Input: part model. Units: mm. Frame: model coordinates. A direction names the side the tool comes from. Give positions to 0.01 mm unless a question says otherwise; leave off trailing zeros. Loops run counter-clockwise (first coordinate to the right, second up) from the corner with the lowest first, then second, coordinate; pieces in that order, holes last. Notation, with made-up numbers: M 7.25,-8 L 22.25,-8 A17 cw 22.25,8 Z; hole C -3,-9 d10. An arc over 180 degrees is marked long. Return JSON: item names as keys, results as strings. Group by question number.
```python
from build123d import *

# Parameters (mm, degrees)
F0_R     = 4.09
F1_DEPTH = 2.6
F2_R     = 5.5
F3_DEPTH = 0.7
F4_R     = 10.95
F5_DEPTH = 1.3
F6_W     = 1.967797
F6_H     = 3.211017
F7_DEPTH = 1


with BuildPart() as f1:
    # F0 (on Top) → F1 (new body)
    with BuildSketch(Plane.XY):
        Circle(F0_R)
    extrude(amount=F1_DEPTH)

    # F2 (on face) → F3 (join)
    with BuildSketch(Plane.XY.offset(2.6)):
        Circle(F2_R)
    extrude(amount=F3_DEPTH)

    # F4 (on face) → F5 (join)
    with BuildSketch(Plane.XY.offset(3.3)):
        Circle(F4_R)
    extrude(amount=F5_DEPTH)

    # F6 (on face) → F7 (cut)
    with BuildSketch(Plane.XY.offset(4.6)):
        Polygon((-9.000013, -5.514394), (-6.681369, -5.514394), (-6.681369, -1.891513), (-4.713572, -1.891513), (-4.713572, -5.514394), (-2.402555, -5.514394), (-2.402555, 5.514419), (-7.222894, 5.514419), (-9.000013, 3.767809), align=None)
        with Locations((-5.69747, 1.811453)):
            Rectangle(F6_W, F6_H, mode=Mode.SUBTRACT)
        Polygon((-1.372894, 5.514419), (-1.372894, -5.514394), (4.172021, -5.514394), (4.172021, -3.424564), (0.938123, -3.424564), (0.938123, 5.514419), align=None)
        Polygon((8.999987, -5.514394), (8.999987, -3.424564), (8.237275, -3.424564), (8.237275, 3.424589), (8.999987, 3.424589), (8.999987, 5.514419), (5.163547, 5.514419), (5.163547, 3.424589), (5.926259, 3.424589), (5.926259, -3.424564), (5.163547, -3.424564), (5.163547, -5.514394), align=None)
    extrude(amount=-F7_DEPTH, mode=Mode.SUBTRACT)


solid = f1.part
```
Item 1: Section A-A, the plane x = 0. Return loops of the section in (y, z).
Item 2: Reachability of faces 1 (the face through (2, 0, 4.6)), 2 (the face through (-5, 3, 3.3)), 3 (the face through (-6, 0.206, 4)) from +Z, -Z, +X, -X, +Y, -Y: full face, straight path, thin tool, end or side. Return the list, or none.
Item 3: Material intervals for line 1 (X direction, y = 2.75, z = 4.15); line 2 (Y direction, x = 5.75, z = 3.9); line 3 (X direction, y = -1.5, z = 3.7), sorted ascending. Write a range as from..to.
Item 4: Section B-B, the plane z = 2. Return loops of the section in (x, y), then the cut area to 3 significant figures.
Item 5: Pull-direction query (X, two-part tool) for faces 4 (the face through (-1.19, -5.37, 2.95)), 5 (the face through (0, 0, 0)), 6 (the face through (1, -5.514, 4)); classes: pulls with the +X half, pulls with the -X half, needs draft (parallel to the pull), parting line crosses it, or undercut.
Item 6: Section D-D, the plane x = -8. Return loops of the section in (y, z), then the cut area to 3 significant figures.
Item 7: Section C-C, the plane y = 2. Return loops of the section in (x, z), then the cut area to 3 significant figures.
Item 8: First-contact query: pin 1 Ø0.5 at (x, z) = (8, 4) entering from -Y; pin 2 Ø0.8 at (x, z) = (5.5, 4) entering from -Y; pin 3 Ø0.5 at (y, z) = (-3.5, 4) entering from +X. Flat tips, straight axial feed; report the tip coordinate or a pass-through.
Answer below:
{
 "1": {"outline": "M -10.95,3.3 L -5.5,3.3 L -5.5,2.6 L -4.09,2.6 L -4.09,0 L 4.09,0 L 4.09,2.6 L 5.5,2.6 L 5.5,3.3 L 10.95,3.3 L 10.95,4.6 L 5.51,4.6 L 5.51,3.6 L -5.51,3.6 L -5.51,4.6 L -10.95,4.6 Z"},
 "2": {"face 1": "+Z, +X, -X, +Y, -Y", "face 2": "-Z", "face 3": "+Z"},
 "3": {"line 1": "-10.6..-9, -6.68..-4.71, -2.4..-1.37, 0.94..5.93, 8.24..10.6", "line 2": "-9.32..-5.51, -3.42..3.42, 5.51..9.32", "line 3": "-10.85..-9, -2.4..-1.37, 0.94..5.93, 8.24..10.85"},
 "4": {"outline": "C 0,0 d8.18", "area": "52.6 mm^2"},
 "5": {"face 4": "parting line crosses it", "face 5": "needs draft", "face 6": "undercut"},
 "6": {"outline": "M -7.48,3.3 L 7.48,3.3 L 7.48,4.6 L 4.75,4.6 L 4.75,3.6 L -5.51,3.6 L -5.51,4.6 L -7.48,4.6 Z", "area": "9.17 mm^2"},
 "7": {"outline": "M -10.77,3.3 L -5.12,3.3 L -5.12,2.6 L -3.57,2.6 L -3.57,0 L 3.57,0 L 3.57,2.6 L 5.12,2.6 L 5.12,3.3 L 10.77,3.3 L 10.77,4.6 L 8.24,4.6 L 8.24,3.6 L 5.93,3.6 L 5.93,4.6 L 0.94,4.6 L 0.94,3.6 L -1.37,3.6 L -1.37,4.6 L -2.4,4.6 L -2.4,3.6 L -4.71,3.6 L -4.71,4.6 L -6.68,4.6 L -6.68,3.6 L -9,3.6 L -9,4.6 L -10.77,4.6 Z", "area": "44.5 mm^2"},
 "8": {"pin 1": "y = -7.74", "pin 2": "y = -9.69", "pin 3": "x = 10.46"}
}
